from build123d import *

# Parameters (mm, degrees)
SKETCH1_W           = 2
SKETCH1_H           = 20
BOSS_EXTRUDE1_DEPTH = 2
CUT_EXTRUDE1_DEPTH  = 110.326849401


with BuildPart() as part:
    # Sketch1 → Boss-Extrude1 (new body)
    with BuildSketch(Plane.XY):
        with BuildLine():
            Line((16.5, 0), (0, 0))
            Line((0, 0), (0, 92))
            Line((0, 92), (16.5, 92))
            Line((16.5, 92), (16.5, 94))
            Line((16.5, 94), (15.9, 94))
            ThreePointArc((15.9, 94), (15.864589803, 94.15), (15.9, 94.3))
            Line((15.9, 94.3), (16.5, 95.5))
            ThreePointArc((16.5, 95.5), (16.566697747, 95.572982477), (16.661803399, 95.6))
            Line((16.661803399, 95.6), (36.338196601, 95.6))
            ThreePointArc((36.338196601, 95.6), (36.433302253, 95.572982477), (36.5, 95.5))
            Line((36.5, 95.5), (37.1, 94.3))
            ThreePointArc((37.1, 94.3), (37.135410197, 94.15), (37.1, 94))
            Line((37.1, 94), (36.5, 94))
            Line((36.5, 94), (36.5, 92))
            Line((36.5, 92), (53, 92))
            Line((53, 92), (53, 0))
            Line((53, 0), (36.5, 0))
            Line((36.5, 0), (36.5, -2))
            Line((36.5, -2), (37.1, -2))
            ThreePointArc((37.1, -2), (37.135410197, -2.15), (37.1, -2.3))
            Line((37.1, -2.3), (36.5, -3.5))
            ThreePointArc((36.5, -3.5), (36.433302253, -3.572982477), (36.338196601, -3.6))
            Line((36.338196601, -3.6), (16.661803399, -3.6))
            ThreePointArc((16.661803399, -3.6), (16.566697747, -3.572982477), (16.5, -3.5))
            Line((16.5, -3.5), (15.9, -2.3))
            ThreePointArc((15.9, -2.3), (15.864589803, -2.15), (15.9, -2))
            Line((15.9, -2), (16.5, -2))
            Line((16.5, -2), (16.5, 0))
        make_face()
        with Locations((3, 68)):
            Rectangle(SKETCH1_W, SKETCH1_H, mode=Mode.SUBTRACT)
        with Locations((50, 68)):
            Rectangle(SKETCH1_W, SKETCH1_H, mode=Mode.SUBTRACT)
        with Locations((50, 24)):
            Rectangle(SKETCH1_W, SKETCH1_H, mode=Mode.SUBTRACT)
        with Locations((3, 24)):
            Rectangle(SKETCH1_W, SKETCH1_H, mode=Mode.SUBTRACT)
    extrude(amount=BOSS_EXTRUDE1_DEPTH)

    # Sketch2 → Cut-Extrude1 (cut, through all)
    with BuildSketch(Plane.XY.offset(2)):
        Polygon((16.344420914, 16), (18.076471722, 19), (16.344420914, 22), (12.880319299, 22), (11.148268492, 19), (12.880319299, 16), align=None)
        Polygon((20.674547933, 26.5), (18.942497126, 23.5), (20.674547933, 20.5), (24.138649548, 20.5), (25.870700356, 23.5), (24.138649548, 26.5), align=None)
        Polygon((12.880319299, 25), (16.344420914, 25), (18.076471722, 28), (16.344420914, 31), (12.880319299, 31), (11.148268492, 28), align=None)
        Polygon((20.674547933, 35.5), (18.942497126, 32.5), (20.674547933, 29.5), (24.138649548, 29.5), (25.870700356, 32.5), (24.138649548, 35.5), align=None)
        Polygon((12.880319299, 40), (11.148268492, 37), (12.880319299, 34), (16.344420914, 34), (18.076471722, 37), (16.344420914, 40), align=None)
        Polygon((20.674547933, 44.5), (18.942497126, 41.5), (20.674547933, 38.5), (24.138649548, 38.5), (25.870700356, 41.5), (24.138649548, 44.5), align=None)
        Polygon((12.880319299, 49), (11.148268492, 46), (12.880319299, 43), (16.344420914, 43), (18.076471722, 46), (16.344420914, 49), align=None)
        Polygon((12.880319299, 52), (16.344420914, 52), (18.076471722, 55), (16.344420914, 58), (12.880319299, 58), (11.148268492, 55), align=None)
        Polygon((20.674547933, 62.5), (18.942497126, 59.5), (20.674547933, 56.5), (24.138649548, 56.5), (25.870700356, 59.5), (24.138649548, 62.5), align=None)
        Polygon((12.880319299, 67), (11.148268492, 64), (12.880319299, 61), (16.344420914, 61), (18.076471722, 64), (16.344420914, 67), align=None)
        Polygon((20.674547933, 71.5), (18.942497126, 68.5), (20.674547933, 65.5), (24.138649548, 65.5), (25.870700356, 68.5), (24.138649548, 71.5), align=None)
        Polygon((12.880319299, 76), (11.148268492, 73), (12.880319299, 70), (16.344420914, 70), (18.076471722, 73), (16.344420914, 76), align=None)
        Polygon((24.138649548, 47.5), (25.870700356, 50.5), (24.138649548, 53.5), (20.674547933, 53.5), (18.942497126, 50.5), (20.674547933, 47.5), align=None)
        Polygon((31.932878182, 16), (33.66492899, 19), (31.932878182, 22), (28.468776567, 22), (26.73672576, 19), (28.468776567, 16), align=None)
        Polygon((36.263005201, 26.5), (34.530954394, 23.5), (36.263005201, 20.5), (39.727106816, 20.5), (41.459157624, 23.5), (39.727106816, 26.5), align=None)
        Polygon((28.468776567, 25), (31.932878182, 25), (33.66492899, 28), (31.932878182, 31), (28.468776567, 31), (26.73672576, 28), align=None)
        Polygon((36.263005201, 35.5), (34.530954394, 32.5), (36.263005201, 29.5), (39.727106816, 29.5), (41.459157624, 32.5), (39.727106816, 35.5), align=None)
        Polygon((28.468776567, 40), (26.73672576, 37), (28.468776567, 34), (31.932878182, 34), (33.66492899, 37), (31.932878182, 40), align=None)
        Polygon((36.263005201, 44.5), (34.530954394, 41.5), (36.263005201, 38.5), (39.727106816, 38.5), (41.459157624, 41.5), (39.727106816, 44.5), align=None)
        Polygon((28.468776567, 49), (26.73672576, 46), (28.468776567, 43), (31.932878182, 43), (33.66492899, 46), (31.932878182, 49), align=None)
        Polygon((28.468776567, 52), (31.932878182, 52), (33.66492899, 55), (31.932878182, 58), (28.468776567, 58), (26.73672576, 55), align=None)
        Polygon((36.263005201, 62.5), (34.530954394, 59.5), (36.263005201, 56.5), (39.727106816, 56.5), (41.459157624, 59.5), (39.727106816, 62.5), align=None)
        Polygon((28.468776567, 67), (26.73672576, 64), (28.468776567, 61), (31.932878182, 61), (33.66492899, 64), (31.932878182, 67), align=None)
        Polygon((36.263005201, 71.5), (34.530954394, 68.5), (36.263005201, 65.5), (39.727106816, 65.5), (41.459157624, 68.5), (39.727106816, 71.5), align=None)
        Polygon((28.468776567, 76), (26.73672576, 73), (28.468776567, 70), (31.932878182, 70), (33.66492899, 73), (31.932878182, 76), align=None)
        Polygon((39.727106816, 47.5), (41.459157624, 50.5), (39.727106816, 53.5), (36.263005201, 53.5), (34.530954394, 50.5), (36.263005201, 47.5), align=None)
    extrude(amount=-CUT_EXTRUDE1_DEPTH, mode=Mode.SUBTRACT)


solid = part.part
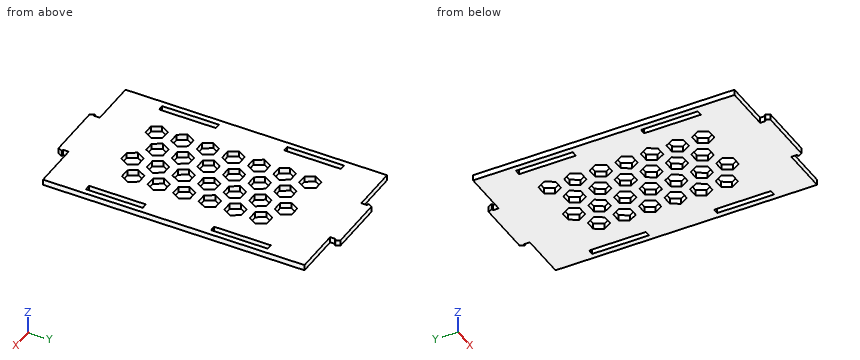
Can you work these out from the model? Positions are in its coordinate system, mm. Give positions to 0.01 mm unless a question says otherwise; leave off trailing zeros. Loops run counter-clockwise (first coordinate to the right, second up) from the corner with the lowest first, then second, coordinate; pieces in that order, holes last. Notation, with made-up numbers: (-20.75, 21) - (-5.75, 21) arc R23 cw to (-5.75, 53) - close; hole circle Ø1 at (-29, 57). An arc over 180 degrees is marked (long way). Answer as a JSON object with one key per item and string values.
Q1. Imagine slicing it at B-B on z = 1.05. Give the number of separate pieces and of enclosed holes in the cut face, plus the area to 3 significant figures.
Geometry says:
{"separate pieces": "1", "enclosed holes": "30", "area": "4,050 mm²"}
Q2. Will these pins go through, and if not, where does the flat tip stop? P1, Ø0.6, axis at y = -1.5, z = 1, coming from the +X side; P2, Ø0.6, axis at y = -0.5, z = 1, coming from the -X side; P3, Ø1, axis at x = 43, z = 0.5, coming from the +Y side.
Geometry says:
{"P1": "x = 36.5", "P2": "x = 16.5", "P3": "y = 92"}
Q3. Imagine slicing it at C-C on x = 8. Write out the boundary of the cut face in (y, z), plus the area to 3 significant figures.
Geometry says:
{"outline": "(0, 0) - (92, 0) - (92, 2) - (0, 2) - close", "area": "184 mm²"}
Q4. If I drill on L1, parallel to X at y = 28, z = 0.65; L2, parallel to X at y = 77, z = 1.3; L3, parallel to X at y = 36.5, z = 1.2, over which ranges is the centre line in solid material (lowest first)?
Geometry says:
{"L1": "0 to 2, 4 to 11.15, 18.08 to 26.74, 33.66 to 49, 51 to 53", "L2": "0 to 2, 4 to 49, 51 to 53", "L3": "0 to 11.44, 17.79 to 27.03, 33.38 to 53"}
Q5. Imagine slicing it at A-A on x = 22. Write out the boundary of the cut face in (y, z), plus the area to 3 significant figures.
Geometry says:
{"outline": "(-3.6, 0) - (20.5, 0) - (20.5, 2) - (-3.6, 2) - close; (26.5, 0) - (29.5, 0) - (29.5, 2) - (26.5, 2) - close; (35.5, 0) - (38.5, 0) - (38.5, 2) - (35.5, 2) - close; (44.5, 0) - (47.5, 0) - (47.5, 2) - (44.5, 2) - close; (53.5, 0) - (56.5, 0) - (56.5, 2) - (53.5, 2) - close; (62.5, 0) - (65.5, 0) - (65.5, 2) - (62.5, 2) - close; (71.5, 0) - (95.6, 0) - (95.6, 2) - (71.5, 2) - close", "area": "126 mm²"}
